```python
from build123d import *

# Parameters (mm, degrees)
F0_W      = 71
F0_H      = 40
F1_DEPTH  = 3
F2_W      = 5
F2_H      = 40
F3_DEPTH  = 40
F4_R      = 1
F5_DEPTH  = 3.001
F7_DEPTH  = 62.001
F13_DEPTH = 2.5
F14_R     = 8
F15_R     = 2


with BuildPart() as f1:
    # F0 (on Top) → F1 (new body)
    with BuildSketch(Plane.XY):
        with Locations((35.5, -20)):
            Rectangle(F0_W, F0_H)
    extrude(amount=F1_DEPTH)

    # F2 (on face) → F3 (join)
    with BuildSketch(Plane.XY.offset(3)):
        with Locations((11.5, -20)):
            Rectangle(F2_W, F2_H)
        with Locations((59.5, -20)):
            Rectangle(F2_W, F2_H)
    extrude(amount=F3_DEPTH)

    # F4 (on face) → F5 (cut, through all)
    with BuildSketch(Plane.XY.offset(3)):
        with Locations((4.5, -6)):
            Circle(F4_R)
        with Locations((4.5, -34)):
            Circle(F4_R)
        with Locations((66.5, -6)):
            Circle(F4_R)
        with Locations((66.5, -34)):
            Circle(F4_R)
    extrude(amount=-F5_DEPTH, mode=Mode.SUBTRACT)

    # F6 (on face) → F7 (cut, through all)
    with BuildSketch(Plane(origin=(9, 0, 0), x_dir=(0, -1, 0), z_dir=(-1, 0, 0))):
        Polygon((10, 17.6602540378), (5, 9), (15, 9), align=None)
        Polygon((25, 28.3397459622), (20, 37), (15, 28.3397459622), align=None)
        Polygon((35, 9), (30, 17.6602540378), (25, 9), align=None)
    extrude(amount=-F7_DEPTH, mode=Mode.SUBTRACT)

    # F12 (on 3pt) → F13 (join, symmetric)
    with BuildSketch(Plane.XZ.offset(20)):
        Polygon((62, 28.3397459622), (62, 3), (71, 3), align=None)
        Polygon((0, 3), (9, 3), (9, 28.3397459622), align=None)
    extrude(amount=F13_DEPTH, both=True)

    # F14
    f14_edges = [f1.edges().sort_by_distance(p)[0] for p in [
        (71, 0, 1.5),
        (0, 0, 1.5),
        (71, -40, 1.5),
        (0, -40, 1.5),
    ]]
    fillet(f14_edges, radius=F14_R)

    # F15
    f15_edges = [f1.edges().sort_by_distance(p)[0] for p in [
        (9, -40, 23),
        (9, 0, 23),
        (62, -40, 23),
        (62, 0, 23),
        (4.5, -17.5, 15.669873),
        (4.5, -22.5, 15.669873),
        (66.5, -17.5, 15.669873),
        (66.5, -22.5, 15.669873),
        (57, 0, 23),
        (14, 0, 23),
        (57, -40, 23),
        (14, -40, 23),
    ]]
    fillet(f15_edges, radius=F15_R)


solid = f1.part
```
Source: CAD feature listing. Evaluate the final solid. Frame: model axes, mm. A direction names the side the tool comes from. Give positions to 0.01 mm unless a question says otherwise; leave off trailing zeros. Loops run counter-clockwise (first coordinate to the right, second up) from the corner with the lowest first, then second, coordinate; pieces in that order, holes last. Notation, with made-up numbers: (55.5, 42.25) - (76.5, 42.25) arc R12 ccw to (76.5, 63.25) - close; hole circle Ø5 at (33.5, 53). An arc over 180 degrees is marked (long way). Use CSV: the item, a comma, the result in double quotes.
1) Line query: line 1 (X direction, y = -27.5, z = 28); line 2 (Y direction, x = 4.5, z = 1.65); line 3 (Y direction, x = 66, z = 2). Output: solid intervals per line, ascending.
Worked out:
line 1,"x = 9 to 14, 57 to 62"
line 2,"y = -39.19 to -35, -33 to -7, -5 to -0.81"
line 3,"y = -39.42 to -34.87, -33.13 to -6.87, -5.13 to -0.58"
2) Cut plane B-B (y = -28.5). Output: boundary loops of the cut face in (x, z).
Worked out:
outline,"(0, 0) - (71, 0) - (71, 3) - (62, 3) - (62, 9) - (57, 9) - (57, 3) - (14, 3) - (14, 9) - (9, 9) - (9, 3) - (0, 3) - close; (9, 15.06) - (14, 15.06) - (14, 43) - (9, 43) - close; (57, 15.06) - (62, 15.06) - (62, 43) - (57, 43) - close"
3) Set-up query: faces 4 (the flat face through (67, -30, 3)), 5 (the flat face through (11.465, -12.535, 13.27)), 6 (the flat face through (14, -20, 23)). Return all of +Z, -Z, +X, -X, +Y, -Y with unobstructed straight access to the full face (end or side cutting, diameter ignored); none if empty.
Worked out:
face 4,"+Z, +X, -Y"
face 5,"+X, -X"
face 6,"+Z, +Y, -Y"
4) Cut plane D-D (y = -34). Output: boundary loops of the cut face in (x, z), and give its area (3 significant figures).
Worked out:
outline,"(0.25, 0) - (3.5, 0) - (3.5, 3) - (0.25, 3) - close; (5.5, 0) - (65.5, 0) - (65.5, 3) - (62, 3) - (62, 9) - (57, 9) - (57, 3) - (14, 3) - (14, 9) - (9, 9) - (9, 3) - (5.5, 3) - close; (9, 10.73) - (14, 10.73) - (14, 43) - (9, 43) - close; (57, 10.73) - (62, 10.73) - (62, 43) - (57, 43) - close; (67.5, 0) - (70.75, 0) - (70.75, 3) - (67.5, 3) - close"
area,"582 mm^2"
5) Pin query (flat end, axial travel): P1, Ø1.5, axis at x = 56, z = 10.5, coming from the -Y side; P2, Ø7.5, axis at x = 5.5, z = 16.5, coming from the -Y side; P3, Ø2, axis at x = 4.5, z = 12, coming from the +Y side; P4, Ø2.5, axis at x = 66.5, y = -34, coming from the +Z side. Return the tip coordinate at first contact, or that it passes through.
Worked out:
P1,"passes through"
P2,"stops at y = -38.97"
P3,"stops at y = -17.5"
P4,"stops at z = 3"
6) Cut plane C-C (x = 58). Output: boundary loops of the cut face in (y, z).
Worked out:
outline,"(-40, 0) - (0, 0) - (0, 3) - (-0.27, 3) - (-0.27, 43) - (-39.73, 43) - (-39.73, 3) - (-40, 3) - close; hole (-35, 9) - (-25, 9) - (-30, 17.66) - close; hole (-25, 28.34) - (-15, 28.34) - (-20, 37) - close; hole (-15, 9) - (-5, 9) - (-10, 17.66) - close"
7) Cut plane A-A (z = 34). Output: boundary loops of the cut face in (x, y), and give its area (3 significant figures).
Worked out:
outline,"(9, -38) arc R2 ccw to (11, -40) - (12, -40) arc R2 ccw to (14, -38) - (14, -21.73) - (9, -21.73) - close; (9, -18.27) - (14, -18.27) - (14, -2) arc R2 ccw to (12, 0) - (11, 0) arc R2 ccw to (9, -2) - close; (57, -38) arc R2 ccw to (59, -40) - (60, -40) arc R2 ccw to (62, -38) - (62, -21.73) - (57, -21.73) - close; (57, -18.27) - (62, -18.27) - (62, -2) arc R2 ccw to (60, 0) - (59, 0) arc R2 ccw to (57, -2) - close"
area,"358 mm^2"
8) Mould query, pull axis Y, two halves, no side actions, for faces 1 (the flat face through (7, -22.5, 9)), 2 (the flat face through (59.465, -7.535, 13.391)), 3 (the flat face through (67, -10, 3)). Classes: +Y half, -Y half, draft (parallel to the pull), parting line (faces both ways), or undercut.
Worked out:
face 1,"-Y half"
face 2,"undercut"
face 3,"draft"
